Drawing for the job (mm, zero at the part's lowest x, y, z). Coordinates: 2 decimals unless noted, no trailing zeros. Order: outer loops, then holes, each group sorted by start corner. A loop starts at its lowest first (then second) coordinate and runs counter-clockwise, first axis right, second up.
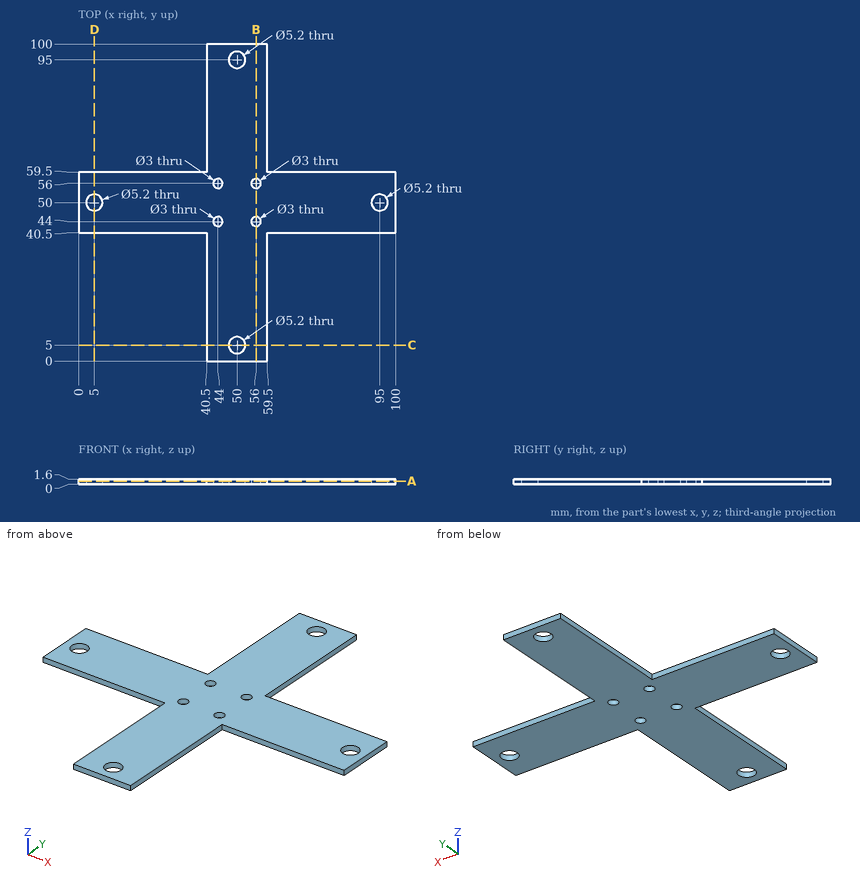
(1) Slice it at A-A, the plane z = 0.9. State how many separate pieces and enclosed holes the cut face has, then the cut area to 3 significant figures.
(2) Probe line 1 (Y direction, x = 50, z = 0.5); line 2 (X direction, y = 95, z = 0.5); line 3 (Y direction, x = 51.5, z = 1). List the from-to ranges inside material, lowest first.
(3) Drop flat-ended pins along their axis: pin 1 (0.5 mm diameter, centred on x = 18, z = 1, fed in from -Y); pin 2 (0.8 mm diameter, centred on x = 21.5, z = 1, fed in from +Y); pin 3 (0.8 mm diameter, centred on y = 20.5, z = 0.5, fed in from -X). Give the stop position or say it passes through.
(4) Slice it at C-C, the plane y = 5. Give the cut face in (x, z).
(5) Slice it at B-B, the plane x = 56. Give the cut face in (y, z), then the cut area to 3 significant figures.
Here are the results:
1. separate pieces: 1
1. enclosed holes: 8
1. area: 3,330 mm2
2. line 1: y = 0 to 2.4, 7.6 to 92.4, 97.6 to 100
2. line 2: x = 40.5 to 47.4, 52.6 to 59.5
2. line 3: y = 0 to 2.88, 7.12 to 92.88, 97.12 to 100
3. pin 1: stops at y = 40.5
3. pin 2: stops at y = 59.5
3. pin 3: stops at x = 40.5
4. outline: (40.5, 0) - (47.4, 0) - (47.4, 1.6) - (40.5, 1.6) - close; (52.6, 0) - (59.5, 0) - (59.5, 1.6) - (52.6, 1.6) - close
5. outline: (0, 0) - (42.5, 0) - (42.5, 1.6) - (0, 1.6) - close; (45.5, 0) - (54.5, 0) - (54.5, 1.6) - (45.5, 1.6) - close; (57.5, 0) - (100, 0) - (100, 1.6) - (57.5, 1.6) - close
5. area: 150 mm2
